Build history of the part. All positions in model axes, mm. Round coordinates to 2 decimals unless told otherwise and drop trailing zeros. Write each loop counter-clockwise with the first axis right and the second up, starting at its lowest first coordinate (ties: lowest second). Pieces come first, ordered by that corner, then holes.
1) Saw through at C-C (y = 333). Write the cut outline in (x, z), plus the area to 3 significant figures.
2) Wall check: probe 1 along Y at (x, z) = (0, -123.5); probe 2 along Y at (x, z) = (0.05, -108.5); probe 3 along Z at (x, y) = (0.05, 177.5). Give the ranges that are in metal, low to high.
3) Saw through at B-B (z = -83.5). Write the cut outline in (x, y), plus the area to 3 significant figures.
from build123d import *

# Parameters (mm, degrees)
BOSS_EXTRUDE1_DEPTH = 0.1016
FILLET1_R           = 25.4
BOSS_EXTRUDE2_DEPTH = 0.2032
FILLET2_R           = 6.35
BOSS_EXTRUDE3_DEPTH = 0.2032


with BuildPart() as part:
    # Sketch1 → Boss-Extrude1 (new body, symmetric)
    with BuildSketch(Plane(origin=(0, 0, 0), x_dir=(0, 0, -1), z_dir=(1, 0, 0))):
        Polygon((0, 0), (0, -112.563749307), (261.582885953, -457.593888215), (450.85, -457.593888215), (450.85, 690.679166755), (208.861297127, 733.352902663), (171.366736958, 520.733599781), (293.482501466, 499.198975136), (217.390599948, 67.706860465), (221.513774593, 49.108421529), align=None)
    extrude(amount=BOSS_EXTRUDE1_DEPTH, both=True)

    # Fillet1
    fillet1_edges = [part.edges().sort_by_distance(p)[0] for p in [
        (0, 499.198975136, -293.482501466),
        (0, 520.733599781, -171.366736958),
        (0, 733.352902663, -208.861297127),
        (0, 690.679166755, -450.85),
        (0, -457.593888215, -450.85),
        (0, -457.593888215, -261.582885953),
        (0, -112.563749307, 0),
    ]]
    fillet(fillet1_edges, radius=FILLET1_R)

    # Sketch5 → Boss-Extrude2 (add)
    with BuildSketch(Plane(origin=(0.1016, 0, 0), x_dir=(0, 0, -1), z_dir=(1, 0, 0))):
        Polygon((24.797918581, 5.497566194), (23.079929145, 13.246915751), (147.069522049, 40.734746721), (148.787511485, 32.985397164), align=None)
    extrude(amount=-BOSS_EXTRUDE2_DEPTH)

    # Fillet2
    fillet2_edges = [part.edges().sort_by_distance(p)[0] for p in [
        (0, 32.985397164, -148.787511485),
        (0, 5.497566194, -24.797918581),
    ]]
    fillet(fillet2_edges, radius=FILLET2_R)

    # Sketch7 → Boss-Extrude3 (add)
    with BuildSketch(Plane(origin=(0.1016, 0, 0), x_dir=(0, 0, -1), z_dir=(1, 0, 0))):
        with BuildLine():
            Line((274.200562117, -465.531388215), (425.45, -465.531388215))
            ThreePointArc((425.45, -465.531388215), (449.023172318, -455.767060533), (458.7875, -432.193888215))
            Line((458.7875, -432.193888215), (458.7875, 669.366434984))
            ThreePointArc((458.7875, 669.366434984), (450.988204091, 690.795131586), (431.239601202, 702.197356752))
            Line((431.239601202, 702.197356752), (235.253809237, 736.758664072))
            ThreePointArc((235.253809237, 736.758664072), (210.34310689, 731.236575989), (196.633286266, 709.717343506))
            Line((196.633286266, 709.717343506), (167.960975549, 547.126111891))
            ThreePointArc((167.960975549, 547.126111891), (173.483063631, 522.215409544), (195.002296115, 508.50558892))
            Line((195.002296115, 508.50558892), (267.089989356, 495.793213726))
            ThreePointArc((267.089989356, 495.793213726), (278.361968276, 488.611879114), (281.254490605, 475.56341598))
            Line((281.254490605, 475.56341598), (209.299504588, 67.530386732))
            Line((209.299504588, 67.530386732), (212.046435601, 55.13978165))
            Line((212.046435601, 55.13978165), (154.818871606, 42.452736156))
            Line((154.818871606, 42.452736156), (153.10088217, 50.202085713))
            Line((153.10088217, 50.202085713), (13.612590153, 19.278275871))
            Line((13.612590153, 19.278275871), (15.330579589, 11.528926315))
            Line((15.330579589, 11.528926315), (-7.9375, 6.37051726))
            Line((-7.9375, 6.37051726), (-7.9375, -104.02374744))
            ThreePointArc((-7.9375, -104.02374744), (-6.199252731, -114.648065445), (-1.165778481, -124.164460435))
            Line((-1.165778481, -124.164460435), (247.634783637, -452.33460121))
            ThreePointArc((247.634783637, -452.33460121), (259.369043538, -462.050461408), (274.200562117, -465.531388215))
        make_face()
    extrude(amount=-BOSS_EXTRUDE3_DEPTH)


solid = part.part
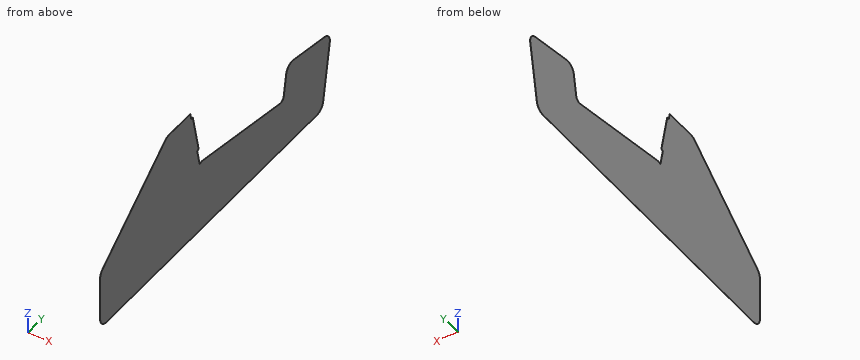
Evaluation:
1. outline: (-0.1, -458.79) - (0.1, -458.79) - (0.1, -256.11) - (-0.1, -256.11) - close
1. area: 41.2 mm2
2. probe 1: y = -288.6 to 43.64
2. probe 2: y = -268.81 to 40.31
2. probe 3: z = -458.79 to -228.69
3. outline: (-0.1, -235.84) - (0.1, -235.84) - (0.1, 34.77) - (-0.1, 34.77) - close
3. area: 55.0 mm2
